Could you check a few things on this drawing? It's one solid part, dimensions in mm from its lowest x, y, z. Give positions to 0.01 mm unless a question says otherwise; leave off trailing zeros. Order: outer loops, then holes, each group sorted by start corner. A loop starts at its lowest first (then second) coordinate and runs counter-clockwise, first axis right, second up. Notation, with made-up numbers: M 66.5,21 L 99.5,21 A20 ccw 99.5,40 Z; hole C -24,-25 d10. An arc over 180 degrees is marked long. Use one line per item in the form item = value. Start each with the question number.
1. I want a section at A-A, the plane z = 5. List the corners of the cut face in (x, y) for me.
2. I need wall thicknesses on L1, parallel to X at y = 9.25, z = 15; L2, parallel to Y at x = 13, z = 15. Which ranges of each line are inside material? Lowest first, please.
3. I want a section at C-C, the plane y = 2.25. List the corners of the cut face in (x, z) for me, and give its area (3 significant figures).
4. I want a section at D-D, the plane z = 3. List the corners of the cut face in (x, y) for me.
5. I want a section at B-B, the plane x = 15. List the corners of the cut face in (y, z) for me.
6. We'd pull the mould along Z, two halves only. Please class the marked faces 1, 2 and 3: +Z half, -Z half, draft (parallel to the pull), parting line (faces both ways), or undercut.
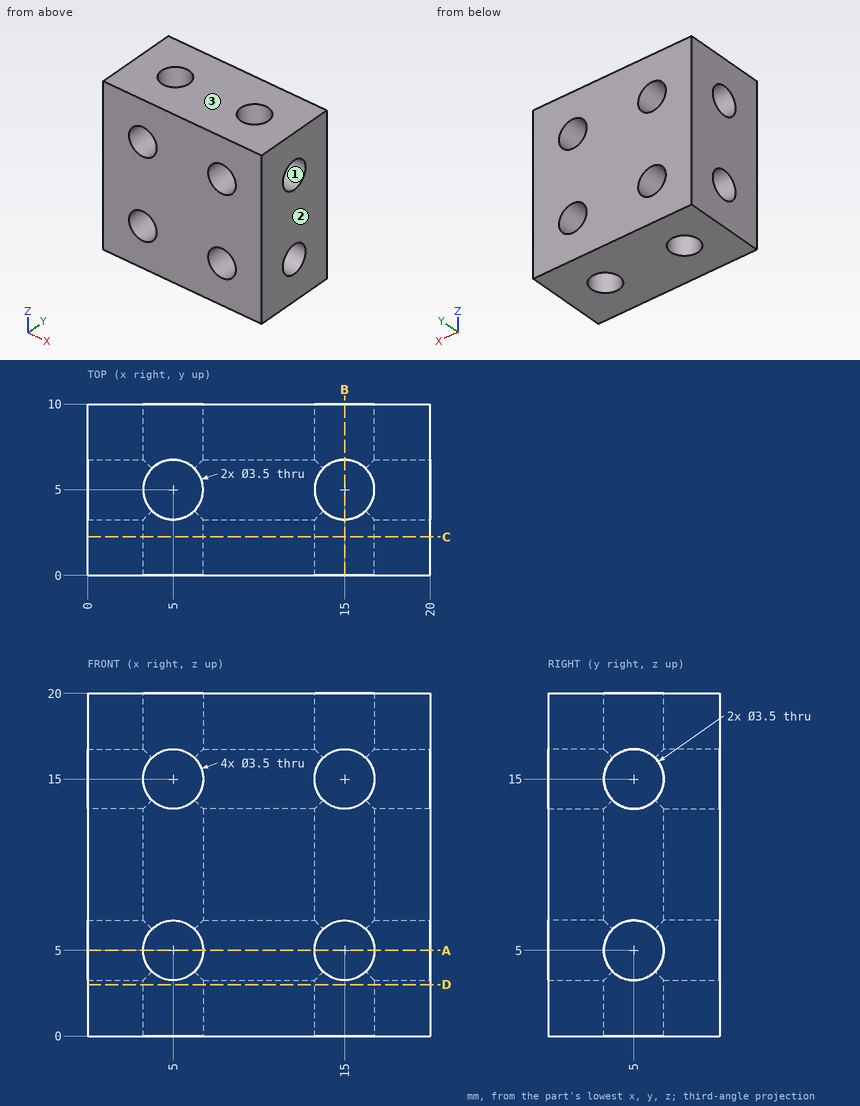
Check result:
q1.outline = M 0,0 L 3.25,0 L 3.25,3.25 L 0,3.25 Z; M 0,6.75 L 3.25,6.75 L 3.25,10 L 0,10 Z; M 6.75,0 L 13.25,0 L 13.25,3.25 L 6.75,3.25 Z; M 6.75,6.75 L 13.25,6.75 L 13.25,10 L 6.75,10 Z; M 16.75,0 L 20,0 L 20,3.25 L 16.75,3.25 Z; M 16.75,6.75 L 20,6.75 L 20,10 L 16.75,10 Z
q2.L1 = 0 to 3.25, 6.75 to 13.25, 16.75 to 20
q2.L2 = 0 to 3.25, 6.75 to 10
q3.outline = M 0,0 L 20,0 L 20,20 L 0,20 Z; hole C 5,5 d3.5; hole C 5,15 d3.5; hole C 15,5 d3.5; hole C 15,15 d3.5
q3.area = 362 mm2
q4.outline = M 0,0 L 20,0 L 20,10 L 0,10 Z; hole C 5,5 d3.5; hole C 15,5 d3.5
q5.outline = M 0,0 L 3.25,0 L 3.25,3.25 L 0,3.25 Z; M 0,6.75 L 3.25,6.75 L 3.25,13.25 L 0,13.25 Z; M 0,16.75 L 3.25,16.75 L 3.25,20 L 0,20 Z; M 6.75,0 L 10,0 L 10,3.25 L 6.75,3.25 Z; M 6.75,6.75 L 10,6.75 L 10,13.25 L 6.75,13.25 Z; M 6.75,16.75 L 10,16.75 L 10,20 L 6.75,20 Z
q6.face_1 = undercut
q6.face_2 = draft
q6.face_3 = +Z half
